Verification items for the finished model (mm, model axes). A direction names the side the tool comes from. Round coordinates to 2 decimals unless told otherwise and drop trailing zeros. Loops run counter-clockwise (first coordinate to the right, second up) from the corner with the lowest first, then second, coordinate; pieces in that order, holes last. Notation, with made-up numbers: (61, -4) - (93, -4) arc R19 cw to (93, 5) - close; hole circle Ø2 at (59.25, -27). An arc over 180 degrees is marked (long way). Use a Markdown table: item, result. Add a question column.
```python
from build123d import *

# Parameters (mm, degrees)
SKETCH1_W           = 75
SKETCH1_H           = 35
BOSS_EXTRUDE1_DEPTH = 10
SKETCH2_R           = 1.8
CUT_EXTRUDE1_DEPTH  = 10
SKETCH3_R           = 1.8
CUT_EXTRUDE2_DEPTH  = 10
SKETCH4_R           = 4
CUT_EXTRUDE4_DEPTH  = 11
FILLET1_R           = 2


with BuildPart() as part:
    # Sketch1 → Boss-Extrude1 (new body)
    with BuildSketch(Plane(origin=(0, 0, 0), x_dir=(1, 0, 0), z_dir=(0, 1, 0))):
        with Locations((37.5, 17.5)):
            Rectangle(SKETCH1_W, SKETCH1_H)
    extrude(amount=BOSS_EXTRUDE1_DEPTH)

    # Sketch2 → Cut-Extrude1 (cut)
    with BuildSketch(Plane.XY):
        with Locations((5, 5)):
            Circle(SKETCH2_R)
        with Locations((37.5, 5)):
            Circle(SKETCH2_R)
        with Locations((70, 5)):
            Circle(SKETCH2_R)
    extrude(amount=-CUT_EXTRUDE1_DEPTH, mode=Mode.SUBTRACT)

    # Sketch3 → Cut-Extrude2 (cut)
    with BuildSketch(Plane(origin=(0, 0, -35), x_dir=(-1, 0, 0), z_dir=(0, 0, -1))):
        with Locations((-5, 5)):
            Circle(SKETCH3_R)
        with Locations((-37.5, 5)):
            Circle(SKETCH3_R)
        with Locations((-70, 5)):
            Circle(SKETCH3_R)
    extrude(amount=-CUT_EXTRUDE2_DEPTH, mode=Mode.SUBTRACT)

    # Sketch4 → Cut-Extrude4 (cut, through all)
    with BuildSketch(Plane.XZ):
        with Locations((12, -9)):
            Circle(SKETCH4_R)
        with Locations((62, -9)):
            Circle(SKETCH4_R)
        with Locations((62, -26)):
            Circle(SKETCH4_R)
        with Locations((12, -26)):
            Circle(SKETCH4_R)
        with BuildLine():
            Line((19, -14.576707994), (55, -14.576707994))
            ThreePointArc((55, -14.576707994), (57.923292006, -17.5), (55, -20.423292006))
            Line((55, -20.423292006), (19, -20.423292006))
            ThreePointArc((19, -20.423292006), (16.076707994, -17.5), (19, -14.576707994))
        make_face()
    extrude(amount=-CUT_EXTRUDE4_DEPTH, mode=Mode.SUBTRACT)

    # Fillet1
    fillet1_edges = [part.edges().sort_by_distance(p)[0] for p in [
        (0, 5, -35),
        (75, 5, -35),
        (75, 5, 0),
        (0, 5, 0),
    ]]
    fillet(fillet1_edges, radius=FILLET1_R)


solid = part.part
```
Q1. Release check for a two-part mould opening along X. For faces 5 (the face through (37, 3, 0)), 6 (the face through (74.4, 5.07, -34.43)), 7 (the face through (68.572, 3.905, -4.93)) record: +X half, -X half, draft (parallel to the pull), parting line (faces both ways), or undercut.
Q2. Set-up check for faces 1 (the face through (38, 5, -25)), 2 (the face through (37, 3, -35)), 3 (the face through (5.831, 3.403, -4.93)), 4 (the face through (37, 5, -20.423)): record each of +Z, -Z, +X, -X, +Y, -Y from which the full face is reachable in a straight line by a thin tool's end or side.
Q3. Section check A-A on z = -17.5. Record the cut outline in (x, y).
Q4. Section check B-B on x = 62. Record the cut outline in (y, z).
Q5. Section check D-D on x = 24. Record the cut outline in (y, z), plus the area to 3 significant figures.
Q6. Go/stop test with flat-tipped pins: pin 1 Ø3 at (x, y) = (70, 5) entering from +Z; pin 2 Ø3 at (x, y) = (5, 5) entering from -Z. Record where each tip stops, or that it passes through.
Q7. Section check C-C on y = 8.5. Record the cut outline in (x, z), plus the area to 3 significant figures.
Q8. Thickness scan on line 1 along Z through (x, y) = (62, 7.25); line 2 along Z through (x, y) = (21.5, 4); line 3 along Y through (x, z) = (37.5, -31.25). Record the ranges inside material, lowest first.
Determined:
| question | item | result |
|---|---|---|
| 1 | face 5 | draft |
| 1 | face 6 | +X half |
| 1 | face 7 | undercut |
| 2 | face 1 | -Z |
| 2 | face 2 | -Z, +X, -X, +Y, -Y |
| 2 | face 3 | +Z |
| 2 | face 4 | +Y, -Y |
| 3 | outline | (0, 0) - (16.08, 0) - (16.08, 10) - (0, 10) - close; (57.92, 0) - (75, 0) - (75, 10) - (57.92, 10) - close |
| 4 | outline | (0, -35) - (10, -35) - (10, -30) - (0, -30) - close; (0, -22) - (10, -22) - (10, -13) - (0, -13) - close; (0, -5) - (10, -5) - (10, 0) - (0, 0) - close |
| 5 | outline | (0, -35) - (10, -35) - (10, -20.42) - (0, -20.42) - close; (0, -14.58) - (10, -14.58) - (10, 0) - (0, 0) - close |
| 5 | area | 292 mm² |
| 6 | pin 1 | stops at z = -10 |
| 6 | pin 2 | stops at z = -25 |
| 7 | outline | (0, -33) arc R2 ccw to (2, -35) - (73, -35) arc R2 ccw to (75, -33) - (75, -2) arc R2 ccw to (73, 0) - (2, 0) arc R2 ccw to (0, -2) - close; hole circle Ø8 at (12, -26); hole circle Ø8 at (12, -9); hole (19, -20.42) - (55, -20.42) arc R2.92 ccw to (55, -14.58) - (19, -14.58) arc R2.92 ccw to start; hole circle Ø8 at (62, -26); hole circle Ø8 at (62, -9) |
| 7 | area | 2,180 mm² |
| 8 | line 1 | z = -35 to -30, -22 to -13, -5 to 0 |
| 8 | line 2 | z = -35 to -20.42, -14.58 to 0 |
| 8 | line 3 | y = 0 to 3.2, 6.8 to 10 |
